Work out the finished part from the listing and answer in its coordinate system (mm). Face numbers are marked on the shaded views. A direction names the side the tool comes from. Coordinates: 2 decimals unless noted, no trailing zeros. Order: outer loops, then holes, each group sorted by start corner. A loop starts at its lowest first (then second) coordinate and runs counter-clockwise, first axis right, second up.
1. The part is cut by section B-B, the plane y = 4.5. Give the vertices of the cut face in (x, z), then the cut area to 3 significant figures.
2. Determine the mould class of the marked faces 4, 5, 6 and 7 for opening direction Z: +Z half, -Z half, draft (parallel to the pull), parting line (faces both ways), or undercut.
3. A flat-ended cylindrical pin translates along its axis: pin 1 Ø0.8 at (x, y) = (-13.5, 2) entering from -Z. Find the tip coordinate at first contact, or state that the pin passes through.
4. Find the intervals of material crossed by probe 1 along X at (y, z) = (3.5, -14); probe 2 along X at (y, z) = (1.75, -1.5), in increasing order.
5. A tool of negligible diameter and unlimited length cuts with its end or side. For the marked faces 1, 2 and 3, from which of +Z, -Z, +X, -X, +Y, -Y can it reach the whole face along a straight path? Write none if from no direction.
6. The part is cut by section A-A, the plane x = 0. Give the vertices of the cut face in (y, z), then the cut area to 3 significant figures.
7. The part is cut by section D-D, the plane x = 13. Give the vertices of the cut face in (y, z), then the cut area to 3 significant figures.
8. The part is cut by section C-C, the plane z = -2. Give the vertices of the cut face in (x, y).
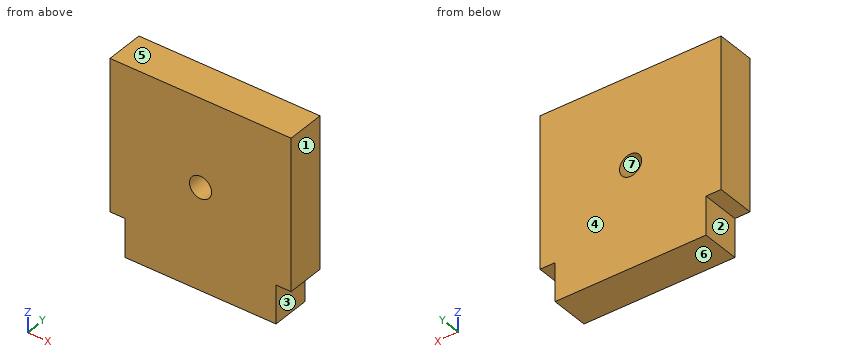
```python
from build123d import *

# Parameters (mm, degrees)
BOSS_EXTRUDE1_DEPTH   = 6.35
F_6_CLEARANCE_HOLE1_D = 3.6576


with BuildPart() as part:
    # Sketch1 → Boss-Extrude1 (new body)
    with BuildSketch(Plane(origin=(0, 0, 0), x_dir=(1, 0, 0), z_dir=(0, 1, 0))):
        Polygon((-12.5, 12.5), (-15, 12.5), (-15, -12.5), (15, -12.5), (15, 12.5), (12.5, 12.5), (12.5, 18.85), (-12.5, 18.85), align=None)
    extrude(amount=BOSS_EXTRUDE1_DEPTH)

    # #6 Clearance Hole1 (through all)
    with Locations(Plane(origin=(0, 6.35, -2.0352), x_dir=(0, 0, 1), z_dir=(0, 1, 0))):
        with Locations((0, 0)):
            Hole(F_6_CLEARANCE_HOLE1_D / 2)


solid = part.part
```
Geometry says:
1. outline: (-15, -12.5) - (-12.5, -12.5) - (-12.5, -18.85) - (12.5, -18.85) - (12.5, -12.5) - (15, -12.5) - (15, 12.5) - (-15, 12.5) - close; hole circle Ø3.66 at (0, -2.04)
1. area: 898 mm2
2. face 4: draft
2. face 5: +Z half
2. face 6: -Z half
2. face 7: undercut
3. pin 1: stops at z = -12.5
4. probe 1: x = -12.5 to 12.5
4. probe 2: x = -15 to -1.75, 1.75 to 15
5. face 1: +Z, -Z, +X, +Y, -Y
5. face 2: -Z, -X, +Y, -Y
5. face 3: -Z, +X, +Y, -Y
6. outline: (0, -18.85) - (6.35, -18.85) - (6.35, -3.86) - (0, -3.86) - close; (0, -0.21) - (6.35, -0.21) - (6.35, 12.5) - (0, 12.5) - close
6. area: 176 mm2
7. outline: (0, -12.5) - (6.35, -12.5) - (6.35, 12.5) - (0, 12.5) - close
7. area: 159 mm2
8. outline: (-15, 0) - (-1.83, 0) - (-1.83, 6.35) - (-15, 6.35) - close; (1.83, 0) - (15, 0) - (15, 6.35) - (1.83, 6.35) - close
